The listing builds one solid part. Answer for the finished solid, in the listing's coordinates (mm). A direction names the side the tool comes from. Give positions to 0.01 mm unless a question says otherwise; leave off trailing zeros. Loops run counter-clockwise (first coordinate to the right, second up) from the corner with the lowest first, then second, coordinate; pieces in that order, holes last.
Item 1: Each of these flat-tipped pins is pushed along its axis until it touches: pin 1 Ø5 at (x, z) = (-10, 6.5) entering from -Y; pin 2 Ø3.5 at (y, z) = (3.175, 6.35) entering from +X. Where does it stop, or does it pass through?
Item 2: Section C-C, the plane z = 4 is taken. Give the vertices of the cut face in (x, y) (3 decimals), and give its area (3 significant figures).
Item 3: A tool of negligible diameter and unlimited length cuts with its end or side. For faces 5 (the face through (-9, 12.7, 6)), 6 (the face through (-21, 0, 6)), from which of +Z, -Z, +X, -X, +Y, -Y can it reach the whole face along a straight path? Write none if from no direction.
Item 4: Section A-A, the plane z = 6.35 is taken. Give the number of separate pieces and of enclosed holes in the cut face, and give its area (3 significant figures).
Item 5: Consider line 1 along X through (y, z) = (4.5, 1.5) (3 decimals); line 2 along Y through (x, z) = (-20.5, 6.35); line 3 along X through (y, z) = (17.25, 6.35) (3 decimals). Determine where each line is inside the solid, lowest interval first.
Item 6: Section B-B, the plane y = 9.75 is taken. Give the vertices of the cut face in (x, z) (3 decimals), and give its area (3 significant figures).
Item 7: The mould has two halves that part along Z. Classify faces 1 (the face through (-13.185, 15.919, 5.072)), 2 (the face through (-10, 14, 0)), 3 (the face through (-20.615, 4.514, 5.497)), 4 (the face through (-10, 19.05, 6)): pulls with the +Z half, pulls with the -Z half, needs draft (parallel to the pull), parting line crosses it, or undercut.
Autodesk Inventor part; units mm, degrees
ref_plane "YZ Plane" through (0, 0, 0) normal (1, 0, 0) x (0, 1, 0)
ref_plane "XZ Plane" through (0, 0, 0) normal (0, 1, 0) x (-1, 0, 0)
ref_plane "XY Plane" through (0, 0, 0) normal (0, 0, 1) x (1, 0, 0)
sketch "Sketch1" plane through (0, 0, 0) normal (0, 0, 1) x (1, 0, 0)
  line L0 (0, 0) -> (0, 12.7)
  line L1 (0, 12.7) -> (-19.05, 12.7)
  line L2 (-19.05, 12.7) -> (-19.05, 0)
  line L3 (-19.05, 0) -> (-22.225, 0)
  line L4 (-22.225, 0) -> (-22.225, 19.05)
  line L5 (-22.225, 19.05) -> (2.54, 19.05)
  line L6 (2.54, 19.05) -> (2.54, 0)
  line L7 (2.54, 0) -> (0, 0)
  dimension "d0" = 12.7
  dimension "d1" = 19.05
  dimension "d2" = 3.175
  dimension "d4" = 19.05
  dimension "d5" = 24.765
extrude "Extrusion1" add sketch "Sketch1" along normal blind 12.7
sketch "Sketch2" plane through (-22.225, 19.05, 0) normal (0, 1, 0) x (1, 0, 0)
  line L0 (0, 0) -> (0, -12.7)
  line L1 (24.765, 0) -> (24.765, -12.7)
  line L2 (0, -6.35) -> (9.2075, -6.35)
  circle A0 centre (9.2075, -6.35) radius 1.2891
  point P0 (22.225, 0)
  dimension "d8" = 2.5781
extrude "Extrusion2" cut sketch "Sketch2" against normal blind 25.4
sketch "Sketch3" plane through (2.54, 0, 0) normal (1, 0, 0) x (0, 0, -1)
  line L0 (0, 0) -> (-12.7, 0)
  line L1 (-6.35, 0) -> (-6.35, 3.175)
  circle A0 centre (-6.35, 3.175) radius 1.5875
  dimension "d12" = 3.175
  dimension "d14" = 3.175
extrude "Extrusion3" cut sketch "Sketch3" against normal blind 25.4
properties part number "tiny clevis" material "Aluminum 6061"
Worked answers:
1. pin 1: stops at y = 12.7
1. pin 2: stops at x = 2.54
2. outline: (-22.225, 0) - (-19.05, 0) - (-19.05, 12.7) - (0, 12.7) - (0, 0) - (2.54, 0) - (2.54, 19.05) - (-22.225, 19.05) - close
2. area: 230 mm2
3. face 5: +Z, -Z, -Y
3. face 6: +Z, -Z, +X, -X, -Y
4. separate pieces: 4
4. enclosed holes: 0
4. area: 195 mm2
5. line 1: x = -22.225 to -19.05, 0 to 2.54
5. line 2: y = 0 to 1.59, 4.76 to 19.05
5. line 3: x = -22.225 to -14.307, -11.728 to 2.54
6. outline: (-22.225, 0) - (-19.05, 0) - (-19.05, 12.7) - (-22.225, 12.7) - close; (0, 0) - (2.54, 0) - (2.54, 12.7) - (0, 12.7) - close
6. area: 72.6 mm2
7. face 1: undercut
7. face 2: pulls with the -Z half
7. face 3: undercut
7. face 4: needs draft
